Here's how the part is built. I have some questions about the finished solid (model axes, mm). Face numbers are marked on the shaded views. Round coordinates to 2 decimals unless told otherwise and drop trailing zeros. Write each loop counter-clockwise with the first axis right and the second up, starting at its lowest first coordinate (ties: lowest second). Pieces come first, ordered by that corner, then holes. Notation, with made-up numbers: (-32.5, 72.5) -> (-6.5, 72.5) arc R26 ccw to (-6.5, 102.5) -> close; hole circle Ø3 at (13.25, -20.75). An arc over 180 degrees is marked (long way). Answer in a Markdown table with one row per item. Add a question column.
Autodesk Fusion 360 part; units mm, degrees
sketch "Skizze1" plane through (0, 0, 0) normal (0, 0, 1) x (1, 0, 0)
  circle A0 centre (0, 0) radius 13.25
  dimension "d1" = 26.5
extrude "Extrusion1" add sketch "Skizze1" along normal blind 66
sketch "Skizze2" plane through (0, 0, 66) normal (0, 0, 1) x (-1, 0, 0)
  circle A0 centre (0, 0) radius 13.25
  circle A1 centre (0, 0) radius 9
  line L0 (0.75, -14.5) -> (-0.75, -14.5)
  line L1 (-0.75, -14.5) -> (-0.75, -8.5)
  line L2 (-0.75, -8.5) -> (0.75, -8.5)
  line L3 (0.75, -8.5) -> (0.75, -14.5)
  line L4 (12.1824, -7.8995) -> (6.9862, -4.8995)
  line L5 (12.9324, -6.6005) -> (12.1824, -7.8995)
  line L6 (7.7362, -3.6005) -> (12.9324, -6.6005)
  line L7 (6.9862, -4.8995) -> (7.7362, -3.6005)
  line L8 (12.9324, 6.6005) -> (7.7362, 3.6005)
  line L9 (12.1824, 7.8995) -> (12.9324, 6.6005)
  line L10 (6.9862, 4.8995) -> (12.1824, 7.8995)
  line L11 (7.7362, 3.6005) -> (6.9862, 4.8995)
  line L12 (0.75, 14.5) -> (0.75, 8.5)
  line L13 (-0.75, 14.5) -> (0.75, 14.5)
  line L14 (-0.75, 8.5) -> (-0.75, 14.5)
  line L15 (0.75, 8.5) -> (-0.75, 8.5)
  line L16 (-12.1824, 7.8995) -> (-6.9862, 4.8995)
  line L17 (-12.9324, 6.6005) -> (-12.1824, 7.8995)
  line L18 (-7.7362, 3.6005) -> (-12.9324, 6.6005)
  line L19 (-6.9862, 4.8995) -> (-7.7362, 3.6005)
  line L20 (-12.9324, -6.6005) -> (-7.7362, -3.6005)
  line L21 (-12.1824, -7.8995) -> (-12.9324, -6.6005)
  line L22 (-6.9862, -4.8995) -> (-12.1824, -7.8995)
  line L23 (-7.7362, -3.6005) -> (-6.9862, -4.8995)
  dimension "d4" = 18
  dimension "d5" = 1.5
  dimension "d6" = 6
  dimension "d7" = 0.75
  dimension "d8" = 8.5
  dimension "d10" = 360
extrude "Extrusion2" cut sketch "Skizze2" against normal blind 6 contours A0 A1 L8 L10 | A0 A1 L4 L6 | A1 L8 L10 L11 | A1 L1 L2 L3 L4 L6 L7 L8 L10 L11 L12 L14 L15 L16 L18 L19 L20 L22 L23 | A1 L4 L6 L7 | A0 A1 L12 L14 | A0 A1 L1 L3 | A1 L12 L14 L15 | A1 L1 L2 L3 | A0 A1 L16 L18 | A0 A1 L20 L22 | A1 L16 L18 L19 | A1 L20 L22 L23
sketch "Skizze3" plane through (0, 0, 60) normal (0, 0, 1) x (-1, 0, 0)
  arc A0 (-11.8314, -5.9649) -> (-11.0814, -7.2639) centre (0, 0) ccw
  line L0 (-11.0814, -7.2639) -> (-7.3921, -5.1339)
  arc A1 (-7.3921, -5.1339) -> (-0.75, -8.9687) centre (0, 0) ccw
  line L1 (-0.75, -8.9687) -> (-0.75, -13.2288)
  arc A2 (-0.75, -13.2288) -> (0.75, -13.2288) centre (0, 0) ccw
  line L2 (0.75, -13.2288) -> (0.75, -8.9687)
  arc A3 (0.75, -8.9687) -> (7.3921, -5.1339) centre (0, 0) ccw
  line L3 (7.3921, -5.1339) -> (11.0814, -7.2639)
  arc A4 (11.0814, -7.2639) -> (11.8314, -5.9649) centre (0, 0) ccw
  line L4 (11.8314, -5.9649) -> (8.1421, -3.8348)
  arc A5 (8.1421, -3.8348) -> (8.1421, 3.8348) centre (0, 0) ccw
  line L5 (8.1421, 3.8348) -> (11.8314, 5.9649)
  arc A6 (11.8314, 5.9649) -> (11.0814, 7.2639) centre (0, 0) ccw
  line L6 (11.0814, 7.2639) -> (7.3921, 5.1339)
  arc A7 (7.3921, 5.1339) -> (0.75, 8.9687) centre (0, 0) ccw
  line L7 (0.75, 8.9687) -> (0.75, 13.2288)
  arc A8 (0.75, 13.2288) -> (-0.75, 13.2288) centre (0, 0) ccw
  line L8 (-0.75, 13.2288) -> (-0.75, 8.9687)
  arc A9 (-0.75, 8.9687) -> (-7.3921, 5.1339) centre (0, 0) ccw
  line L9 (-7.3921, 5.1339) -> (-11.0814, 7.2639)
  arc A10 (-11.0814, 7.2639) -> (-11.8314, 5.9649) centre (0, 0) ccw
  line L10 (-11.8314, 5.9649) -> (-8.1421, 3.8348)
  arc A11 (-8.1421, 3.8348) -> (-8.1421, -3.8348) centre (0, 0) ccw
  line L11 (-8.1421, -3.8348) -> (-11.8314, -5.9649)
  circle A12 centre (0, 0) radius 4
  dimension "d13" = 8
extrude "Extrusion3" cut sketch "Skizze3" against normal blind 15 contours A12
sketch "Skizze4" plane through (0, 0, 0) normal (0, 0, -1) x (1, 0, 0)
  circle A0 centre (0, 0) radius 13.25
  circle A1 centre (0, 0) radius 3
  line L0 (-1.6583, 2.5) -> (1.6583, 2.5)
  dimension "d16" = 6
  dimension "d17" = 2.5
extrude "Extrusion4" cut sketch "Skizze4" against normal blind 12 contours A1 L0 picked at (0.41, 2.7801)
sketch "Skizze5" plane through (0, -2.5, 0) normal (0, 1, 0) x (-1, 0, 0)
  line L0 (-1.6583, 0) -> (1.6583, 0)
  line L1 (1.6583, 0) -> (1.6583, 12)
  line L2 (1.6583, 12) -> (-1.6583, 12)
  line L3 (-1.6583, 12) -> (-1.6583, 0)
  circle A0 centre (0, 6) radius 2.75
  dimension "d20" = 5.5
  dimension "d21" = 6
extrude "Extrusion5" cut sketch "Skizze5" along normal blind 3 contours L3 A0 | L1 L3 A0 | L1 A0
sketch "Skizze6" plane through (0, -2.5, 0) normal (0, 1, 0) x (-1, 0, 0)
  line L0 (1.6583, 8.1937) -> (1.6583, 12)
  line L1 (1.6583, 12) -> (-1.6583, 12)
  line L2 (-1.6583, 12) -> (-1.6583, 8.1937)
  arc A0 (-1.6583, 8.1937) -> (-1.6583, 3.8063) centre (0, 6) ccw
  line L3 (-1.6583, 3.8063) -> (-1.6583, 0)
  line L4 (-1.6583, 0) -> (1.6583, 0)
  line L5 (1.6583, 0) -> (1.6583, 3.8063)
  arc A1 (1.6583, 3.8063) -> (1.6583, 8.1937) centre (0, 6) ccw
  circle A2 centre (0, 6) radius 2.75
  dimension "d24" = 5.5
extrude "Extrusion6" cut sketch "Skizze6" against normal blind 15 contours A0 A1 A2
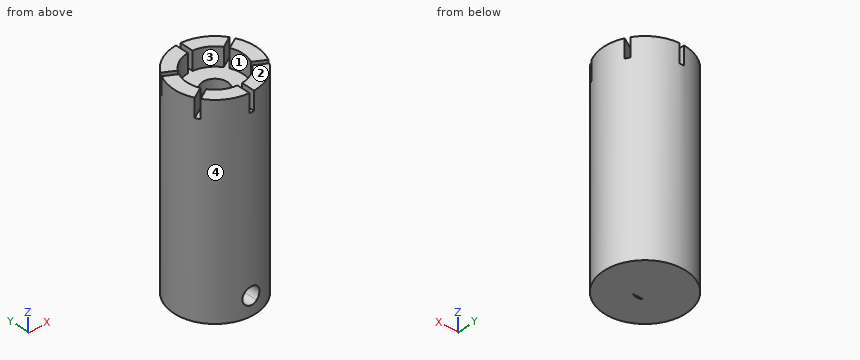
Item 1: For P1, Ø2, axis at y = 11, z = 63, coming from the +X side; P2, Ø2, axis at x = 7.5, z = 40.5, coming from the -Y side; P3, Ø3, axis at x = -9.5, z = 36, coming from the +Y side, each with a flat end and sliding along its axis, tell me the tip position at first contact or that it passes through.
Item 2: If we section it at C-C on z = 56: Please give me the cut outline in (x, y), then the cut area to 3 significant figures.
Item 3: If we section it at D-D on x = 5: Please give me the cut outline in (y, z).
Item 4: If we section it at B-B on y = -1.75: Please give me the cut outline in (x, z).
Item 5: I need wall thicknesses on line 1 along X through (y, z) = (0, 52); line 2 along X through (y, z) = (-0.35, 6); line 3 along Z through (x, y) = (0, -1.25). Which ranges of each line are inside material? Lowest first, please. Write a range as from..to.
Item 6: If we section it at A-A on x = 0: Please give me the cut outline in (y, z), then the cut area to 3 significant figures.
Item 7: If we mould it in two halves opening along Y, with no side actions, what happens to the marked faces 1, 2, 3 and 4? For each: pulls with the +Y half, pulls with the -Y half, needs draft (parallel to the pull), parting line crosses it, or undercut.
Results list:
| question | item | result |
|---|---|---|
| 1 | P1 | x = 8.69 |
| 1 | P2 | y = -11.55 |
| 1 | P3 | y = 10.56 |
| 2 | outline | circle Ø26.5 at (0, 0); hole circle Ø8 at (0, 0) |
| 2 | area | 501 mm² |
| 3 | outline | (-12.27, 0) -> (12.27, 0) -> (12.27, 66) -> (7.48, 66) -> (7.48, 60) -> (-7.48, 60) -> (-7.48, 66) -> (-12.27, 66) -> close |
| 4 | outline | (-13.13, 0) -> (13.13, 0) -> (13.13, 66) -> (8.83, 66) -> (8.83, 60) -> (3.6, 60) -> (3.6, 45) -> (-3.6, 45) -> (-3.6, 60) -> (-8.83, 60) -> (-8.83, 66) -> (-13.13, 66) -> close; hole circle Ø5.5 at (0, 6) |
| 5 | line 1 | -13.25..-4, 4..13.25 |
| 5 | line 2 | -13.25..-2.75, 2.75..13.25 |
| 5 | line 3 | 0..3.25, 8.75..45 |
| 6 | outline | (-13.25, 0) -> (-3, 0) -> (-3, 3.25) -> (-13.25, 3.25) -> close; (-13.25, 8.75) -> (-3, 8.75) -> (-3, 12) -> (-2.5, 12) -> (-2.5, 8.75) -> (0.5, 8.75) -> (0.5, 3.25) -> (-2.5, 3.25) -> (-2.5, 0) -> (13.25, 0) -> (13.25, 60) -> (4, 60) -> (4, 45) -> (-4, 45) -> (-4, 60) -> (-13.25, 60) -> close |
| 6 | area | 1,390 mm² |
| 7 | face 1 | undercut |
| 7 | face 2 | needs draft |
| 7 | face 3 | undercut |
| 7 | face 4 | parting line crosses it |
